Check sheet for the modelled part. Datum: model origin and axes. Units: mm. A direction names the side the tool comes from. Coordinates: 2 decimals unless noted, no trailing zeros. Order: outer loops, then holes, each group sorted by start corner. A loop starts at its lowest first (then second) coordinate and runs counter-clockwise, first axis right, second up.
from build123d import *

# Parameters (mm, degrees)
SKETCH1_R           = 6
BOSS_EXTRUDE1_DEPTH = 7
SKETCH2_R           = 12.5
BOSS_EXTRUDE2_DEPTH = 3
SKETCH3_R           = 12
BOSS_EXTRUDE3_DEPTH = 140.45
SKETCH4_R           = 4.5
CUT_EXTRUDE1_DEPTH  = 152.484991006
LPATTERN1_COUNT     = 2
LPATTERN1_PITCH     = 25


with BuildPart() as part:
    # Sketch1 → Boss-Extrude1 (new body)
    with BuildSketch(Plane.XY):
        Circle(SKETCH1_R)
    extrude(amount=BOSS_EXTRUDE1_DEPTH)

    # Sketch2 → Boss-Extrude2 (add)
    with BuildSketch(Plane.XY.offset(7)):
        Circle(SKETCH2_R)
    extrude(amount=BOSS_EXTRUDE2_DEPTH)

    # Sketch3 → Boss-Extrude3 (add)
    with BuildSketch(Plane.XY.offset(10)):
        with Locations(Location((0, 0, 0), (0, 0, 180))):
            Circle(SKETCH3_R)
    extrude(amount=BOSS_EXTRUDE3_DEPTH)

    # Sketch4 → Cut-Extrude1 (cut, symmetric)
    with BuildSketch(Plane(origin=(0, 0, 0), x_dir=(1, 0, 0), z_dir=(0, 1, 0))):
        with Locations(Location((0, -130.45, 0), (0, 0, 270))):
            Circle(SKETCH4_R)
    cut_extrude1 = extrude(amount=CUT_EXTRUDE1_DEPTH, both=True, mode=Mode.SUBTRACT)

    # LPattern1: Cut-Extrude1 ×2
    with Locations(*[(0, 0, -i * LPATTERN1_PITCH) for i in range(1, LPATTERN1_COUNT)]):
        add(cut_extrude1, mode=Mode.SUBTRACT)


solid = part.part
(1) Cross-section at B-B (y = -2.5). Enter the section's corners in (x, z), and give its area (3 significant figures).
Filled in:
outline: (-12.25, 7) - (-5.45, 7) - (-5.45, 0) - (5.45, 0) - (5.45, 7) - (12.25, 7) - (12.25, 10) - (11.74, 10) - (11.74, 150.45) - (-11.74, 150.45) - (-11.74, 10) - (-12.25, 10) - close; hole circle Ø9 at (0, 105.45); hole circle Ø9 at (0, 130.45)
area: 3,320 mm2
(2) Cross-section at C-C (z = 105.45). Enter the section's corners in (x, y), and give its area (3 significant figures).
Filled in:
outline: (-4.5, -11.12) - (-4.5, 11.12) arc R12 ccw to start; (4.5, -11.12) arc R12 ccw to (4.5, 11.12) - close
area: 242 mm2
(3) Tool access check on faces 5 (the cylindrical face through (-11.446, -3.604, 79.242)), 6 (the flat face through (0, 0, 150.45)), 7 (the flat face through (-3, -5.4, 7)). Record the directions out of +Z, -Z, +X, -X, +Y, -Y that give a thin tool (end or side, any length) a straight path to the whole face; none if there is none.
Filled in:
face 5: +Z
face 6: +Z, +X, -X, +Y, -Y
face 7: -Z
(4) Thickness scan on probe 1 along Z at (x, y) = (0, 4.5); probe 2 along Z at (x, y) = (0, 7.75); probe 3 along X at (y, z) = (0.75, 105.45). Record the ranges inside material, lowest first.
Filled in:
probe 1: z = 0 to 100.95, 109.95 to 125.95, 134.95 to 150.45
probe 2: z = 7 to 100.95, 109.95 to 125.95, 134.95 to 150.45
probe 3: x = -11.98 to -4.5, 4.5 to 11.98
(5) Go/stop test with flat-tipped pins: P1, Ø10.5, axis at x = 0, z = 130.45, coming from the +Y side; P2, Ø12, axis at y = -6, z = 43, coming from the +X side; P3, Ø8, axis at x = 9, z = 29, coming from the -Y side. Record where each tip stops, or that it passes through.
Filled in:
P1: stops at y = 12
P2: stops at x = 12
P3: stops at y = -10.91
(6) Cross-section at D-D (x = -10). Enter the section's corners in (y, z).
Filled in:
outline: (-7.5, 7) - (7.5, 7) - (7.5, 10) - (6.63, 10) - (6.63, 150.45) - (-6.63, 150.45) - (-6.63, 10) - (-7.5, 10) - close
(7) Release check for a two-part mould opening along Z. For faces 1 (the cylindrical face through (-1.72, 0.17, 134.61)), 2 (the cylindrical face through (-6, 0, 3)), 3 (the flat face through (0, 0, 0)), 4 (the flat face through (-7, 10, 10)) record: +Z half, -Z half, draft (parallel to the pull), parting line (faces both ways), or undercut.
Filled in:
face 1: undercut
face 2: draft
face 3: -Z half
face 4: +Z half
(8) Cross-section at A-A (x = 0). Enter the section's corners in (y, z), and give its area (3 significant figures).
Filled in:
outline: (-12.5, 7) - (-6, 7) - (-6, 0) - (6, 0) - (6, 7) - (12.5, 7) - (12.5, 10) - (12, 10) - (12, 100.95) - (-12, 100.95) - (-12, 10) - (-12.5, 10) - close; (-12, 109.95) - (12, 109.95) - (12, 125.95) - (-12, 125.95) - close; (-12, 134.95) - (12, 134.95) - (12, 150.45) - (-12, 150.45) - close
area: 3,100 mm2
